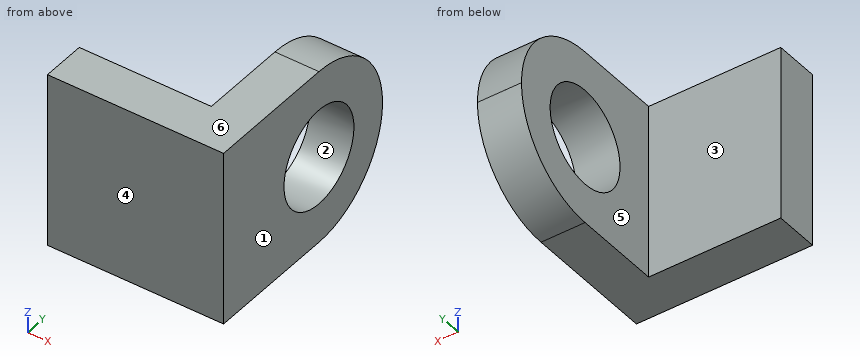
```python
from build123d import *

# Parameters (mm, degrees)
SKETCH1_W           = 20
SKETCH1_H           = 20
BOSS_EXTRUDE1_DEPTH = 5
SKETCH2_W           = 5
SKETCH2_H           = 20
BOSS_EXTRUDE2_DEPTH = 20
SKETCH3_R           = 5.5
CUT_EXTRUDE1_DEPTH  = 34.541019662
FILLET1_R           = 10


with BuildPart() as part:
    # Sketch1 → Boss-Extrude1 (new body)
    with BuildSketch(Plane(origin=(0, 0, 0), x_dir=(1, 0, 0), z_dir=(0, 1, 0))):
        Rectangle(SKETCH1_W, SKETCH1_H)
    extrude(amount=BOSS_EXTRUDE1_DEPTH)

    # Sketch2 → Boss-Extrude2 (add)
    with BuildSketch(Plane(origin=(0, 5, 0), x_dir=(1, 0, 0), z_dir=(0, 1, 0))):
        with Locations((7.5, 0)):
            Rectangle(SKETCH2_W, SKETCH2_H)
    extrude(amount=BOSS_EXTRUDE2_DEPTH)

    # Sketch3 → Cut-Extrude1 (cut, through all)
    with BuildSketch(Plane(origin=(10, 0, 0), x_dir=(0, 0, -1), z_dir=(1, 0, 0))):
        with Locations((0, 15)):
            Circle(SKETCH3_R)
    extrude(amount=-CUT_EXTRUDE1_DEPTH, mode=Mode.SUBTRACT)

    # Fillet1
    fillet1_edges = [part.edges().sort_by_distance(p)[0] for p in [
        (7.5, 25, -10),
        (7.5, 25, 10),
    ]]
    fillet(fillet1_edges, radius=FILLET1_R - 0.0001)  # a hair under: the kernel refuses the full size


solid = part.part
```
Check sheet for the modelled part. Datum: model origin and axes. Units: mm. Face numbers are marked on the shaded views. A direction names the side the tool comes from. Coordinates: 2 decimals unless noted, no trailing zeros. Order: outer loops, then holes, each group sorted by start corner. A loop starts at its lowest first (then second) coordinate and runs counter-clockwise, first axis right, second up. Notation, with made-up numbers: (31, 65) -> (53, 65) arc R26 cw to (53, 102) -> close; hole circle Ø8 at (-10.75, 20.25). An arc over 180 degrees is marked (long way). Write item = value, one per line. Start each with the question number.
1) Mould release check, pull along Y, two halves, no side actions. Record for the marked faces 1, 2, 3 and 4: +Y half, -Y half, draft (parallel to the pull), parting line (faces both ways), or undercut.
2) Cross-section at C-C (z = -2.5). Enter the section's corners in (x, y), then the cut area to 3 significant figures.
3) Material ranges on L1, parallel to Y at x = 8.2, z = 0; L2, parallel to Y at x = -5.5, z = -6.5; L3, parallel to X at y = 16.5, z = -6.75, recorded low to high.
4) Cross-section at D-D (x = -5.5). Enter the section's corners in (y, z), then the cut area to 3 significant figures.
5) Cross-section at B-B (y = 17.75). Enter the section's corners in (x, z), then the cut area to 3 significant figures.
6) Access from +Z, -Z, +X, -X, +Y, -Y to the whole of each face (thin tool, end or side, straight path). Record for the marked faces 5 and 6.
7) Go/stop test with flat-tipped pins: P1, Ø6, axis at y = 18.5, z = 2.5, coming from the -X side; P2, Ø12, axis at x = -2, z = 5, coming from the +Y side. Record where each tip stops, or that it passes through.
Ans:
q1.face_1 = draft
q1.face_2 = undercut
q1.face_3 = +Y half
q1.face_4 = -Y half
q2.outline = (-10, 0) -> (10, 0) -> (10, 10.1) -> (5, 10.1) -> (5, 5) -> (-10, 5) -> close; (5, 19.9) -> (10, 19.9) -> (10, 24.68) -> (5, 24.68) -> close
q2.area = 149 mm²
q3.L1 = 0 to 9.5, 20.5 to 25
q3.L2 = 0 to 5
q3.L3 = 5 to 10
q4.outline = (0, -10) -> (5, -10) -> (5, 10) -> (0, 10) -> close
q4.area = 100 mm²
q5.outline = (5, -9.61) -> (10, -9.61) -> (10, -4.76) -> (5, -4.76) -> close; (5, 4.76) -> (10, 4.76) -> (10, 9.61) -> (5, 9.61) -> close
q5.area = 48.5 mm²
q6.face_5 = +Z, -Z, -X, +Y
q6.face_6 = +Z, +X, -X, +Y, -Y
q7.P1 = 5
q7.P2 = 5
